Input: part model. Units: mm. Frame: model coordinates. A direction names the side the tool comes from. Give positions to 0.01 mm unless a question says otherwise; leave off trailing zeros. Write each loop counter-clockwise with the first axis right and the second up, starting at its lowest first coordinate (ties: lowest second). Pieces come first, ordered by that corner, then holes. Notation, with made-up numbers: (60, 19) - (91, 19) arc R14 cw to (91, 32) - close; hole circle Ø9 at (79, 64.25). An arc over 180 degrees is marked (long way). Answer as CSV lines item,"result". Start each with the question number.
from build123d import *

# Parameters (mm, degrees)
SKETCH_W          = 27
SKETCH_H          = 5
PAD_DEPTH         = 2.5
SKETCH001_R       = 1.7
POCKET_DEPTH      = 13.501
POCKET_DEPTH_BACK = -13.501
SKETCH002_W       = 22
SKETCH002_H       = 3
POCKET001_DEPTH   = 2.5


with BuildPart() as part:
    # Sketch → Pad (new body, symmetric)
    with BuildSketch(Plane.XY):
        Rectangle(SKETCH_W, SKETCH_H)
    extrude(amount=PAD_DEPTH, both=True)

    # Sketch001 → Pocket (cut, two sides)
    with BuildSketch(Plane.YZ) as pocket_sk:
        Circle(SKETCH001_R)
    extrude(amount=-POCKET_DEPTH, mode=Mode.SUBTRACT)
    extrude(pocket_sk.sketch, amount=-POCKET_DEPTH_BACK, mode=Mode.SUBTRACT)

    # Sketch002 → Pocket001 (cut, symmetric)
    with BuildSketch(Plane.XZ):
        with Locations((0, -1.5)):
            Rectangle(SKETCH002_W, SKETCH002_H)
    extrude(amount=POCKET001_DEPTH, both=True, mode=Mode.SUBTRACT)


solid = part.part
1) Reachability of faces 4 (the flat face through (0, 2.5, 1)), 5 (the flat face through (11, 0, -2)) from +Z, -Z, +X, -X, +Y, -Y: full face, straight path, thin tool, end or side. Return the list, or none.
2) Cut plane D-D on x = 3.25. Output: boundary loops of the cut face in (y, z).
3) Cut plane B-B on z = 0.7. Output: boundary loops of the cut face in (x, y), and give its area (3 significant figures).
4) Material intervals for line 1 (X direction, y = 2.3, z = -0.05); line 2 (Z direction, x = -12, y = -1.15); line 3 (Z direction, x = -11.5, y = -1.4), sorted ascending. Write a range as from..to.
5) Cut plane C-C on z = -0.7. Output: boundary loops of the cut face in (x, y), and give its area (3 significant figures).
6) Pull-direction query (Y, two-part tool) for faces 1 (the flat face through (-11, 0, -2)), 2 (the flat face through (0, -2.5, 1)), 3 (the cylindrical face through (0.189, -0.221, 1.686)); classes: +Y half, -Y half, draft (parallel to the pull), parting line (faces both ways), or undercut.
7) Cut plane A-A on y = 0. Output: boundary loops of the cut face in (x, z).
Numbers:
1,face 4,"+Z, -Z, +X, -X, +Y"
1,face 5,"-Z, +Y, -Y"
2,outline,"(-2.5, 0) - (-1.7, 0) arc R1.7 cw to (1.7, 0) - (2.5, 0) - (2.5, 2.5) - (-2.5, 2.5) - close"
3,outline,"(-13.5, -2.5) - (13.5, -2.5) - (13.5, -1.55) - (-13.5, -1.55) - close; (-13.5, 1.55) - (13.5, 1.55) - (13.5, 2.5) - (-13.5, 2.5) - close"
3,area,"51.3 mm²"
4,line 1,"x = -13.5..-11, 11..13.5"
4,line 2,"z = -2.5..-1.25, 1.25..2.5"
4,line 3,"z = -2.5..-0.96, 0.96..2.5"
5,outline,"(-13.5, -2.5) - (-11, -2.5) - (-11, -1.55) - (-13.5, -1.55) - close; (-13.5, 1.55) - (-11, 1.55) - (-11, 2.5) - (-13.5, 2.5) - close; (11, -2.5) - (13.5, -2.5) - (13.5, -1.55) - (11, -1.55) - close; (11, 1.55) - (13.5, 1.55) - (13.5, 2.5) - (11, 2.5) - close"
5,area,"9.51 mm²"
6,face 1,"draft"
6,face 2,"-Y half"
6,face 3,"undercut"
7,outline,"(-13.5, -2.5) - (-11, -2.5) - (-11, -1.7) - (-13.5, -1.7) - close; (-13.5, 1.7) - (13.5, 1.7) - (13.5, 2.5) - (-13.5, 2.5) - close; (11, -2.5) - (13.5, -2.5) - (13.5, -1.7) - (11, -1.7) - close"
